from build123d import *

# Parameters (mm, degrees)
SKIZZE1_W                                   = 27
SKIZZE1_H                                   = 31
AUFSATZ_LINEAR_AUSTRAGEN1_DEPTH             = 20
AUFSATZ_LINEAR_AUSTRAGEN2_DEPTH             = 3
FORMSENKUNG_F_R_M3_SENKSCHRAUBE_MIT_2_COUNT = 2
FORMSENKUNG_F_R_M3_SENKSCHRAUBE_MIT_2_PITCH = 36
SCHNITT_LINEAR_AUSTRAGEN1_DEPTH             = 18
FASE1_SIZE                                  = 5
VERRUNDUNG1_R                               = 2


with BuildPart() as part:
    # Skizze1 → Aufsatz-Linear austragen1 (new body)
    with BuildSketch(Plane.XY):
        Rectangle(SKIZZE1_W, SKIZZE1_H)
    extrude(amount=AUFSATZ_LINEAR_AUSTRAGEN1_DEPTH)

    # Skizze2 → Aufsatz-Linear austragen2 (add)
    with BuildSketch(Plane.XY):
        Polygon((16.25, 17), (-16.25, 17), (-22.25, 9), (-22.25, -9), (-16.25, -17), (16.25, -17), (22.25, -9), (22.25, 9), align=None)
    extrude(amount=-AUFSATZ_LINEAR_AUSTRAGEN2_DEPTH)

    # Skizze3 → Formsenkung für M3 Senkschraube mit Innensechskant1 (revolve, cut)
    with BuildSketch(Plane(origin=(18, 0, -3), x_dir=(0, 1, 0), z_dir=(1, 0, 0))):
        Polygon((0, 0), (0, 3), (1.7, 3), (1.7, 1.77), (3.47, 0), align=None)
    formsenkung_f_r_m3_senkschraube_mit_inne = revolve(axis=Axis((18, 0, -9.35), (0, 0, 1)), mode=Mode.SUBTRACT)

    # Formsenkung f_r M3 Senkschraube mit  2: Formsenkung für M3 Senkschraube mit Innensechskant1 ×2
    with Locations(*[(-i * FORMSENKUNG_F_R_M3_SENKSCHRAUBE_MIT_2_PITCH, 0, 0) for i in range(1, FORMSENKUNG_F_R_M3_SENKSCHRAUBE_MIT_2_COUNT)]):
        add(formsenkung_f_r_m3_senkschraube_mit_inne, mode=Mode.SUBTRACT)

    # Skizze5 → Schnitt-Linear austragen1 (cut)
    with BuildSketch(Plane(origin=(0, 0, -3), x_dir=(-1, 0, 0), z_dir=(0, 0, -1))):
        Polygon((7.25, 14), (-7.25, 14), (-12.25, 9), (-12.25, -2), (12.25, -2), (12.25, 9), align=None)
    extrude(amount=-SCHNITT_LINEAR_AUSTRAGEN1_DEPTH, mode=Mode.SUBTRACT)

    # Fase1
    fase1_edges = [part.edges().sort_by_distance(p)[0] for p in [
        (-13.5, 15.5, 10),
        (13.5, 15.5, 10),
    ]]
    chamfer(fase1_edges, length=FASE1_SIZE)

    # Verrundung1
    verrundung1_edges = [part.edges().sort_by_distance(p)[0] for p in [
        (13.5, -15.5, 10),
        (-13.5, -15.5, 10),
    ]]
    fillet(verrundung1_edges, radius=VERRUNDUNG1_R)


solid = part.part
Design review of the part built by this model. Coordinates are the model's own, in mm. A direction names the side the tool comes from. Coordinates: 2 decimals unless noted, no trailing zeros. Order: outer loops, then holes, each group sorted by start corner. A loop starts at its lowest first (then second) coordinate and runs counter-clockwise, first axis right, second up. Notation, with made-up numbers: M 46.25,-19.5 L 74.25,-19.5 A18 ccw 74.25,8.5 Z; hole C -24,-10 d11. An arc over 180 degrees is marked long. Use a Markdown table: item, result.
(1) Draft analysis for pull direction Y (two halves, no side actions). For faces 5 (the cylindrical face through (12.9, -14.93, 10.14)), 6 (the flat face through (12.25, 4, 6)), 7 (the flat face through (11, 13, 10)), state which applies: released by +Y, released by -Y, zero draft, split by the parting line, or undercut.
Worked answers:
| item | result |
|---|---|
| face 5 | released by -Y |
| face 6 | undercut |
| face 7 | released by +Y |
(2) Add section D-D (y = -10). Give the boundary of the cut face in (x, z), then the cut area to 3 significant figures.
Worked answers:
| item | result |
|---|---|
| outline | M -21.5,-3 L 21.5,-3 L 21.5,0 L 13.5,0 L 13.5,20 L -13.5,20 L -13.5,0 L -21.5,0 Z |
| area | 669 mm2 |
(3) Add section C-C (x = -18). Give the boundary of the cut face in (y, z).
Worked answers:
| item | result |
|---|---|
| outline | M -14.67,-3 L -3.47,-3 L -1.7,-1.23 L -1.7,0 L -14.67,0 Z; M 1.7,-1.23 L 3.47,-3 L 14.67,-3 L 14.67,0 L 1.7,0 Z |
(4) For faces 1 (the flat face through (-12.25, 3, 6)), 2 (the flat face through (0, 15.5, 10)), 3 (the flat face through (-13.5, -2, 10)), 4 (the flat face through (-11, 13, 10)), list the 3-axis set-ups (+Z, -Z, +X, -X, +Y, -Y) from which the entire face can be reached by the end or side of a thin tool; tool diameter is ignored.
Worked answers:
| item | result |
|---|---|
| face 1 | -Z |
| face 2 | +Z, +X, -X, +Y |
| face 3 | +Z, -X, +Y, -Y |
| face 4 | +Z, -X, +Y |
(5) Add section A-A (y = 0). Give the boundary of the cut face in (x, z), then the cut area to 3 significant figures.
Worked answers:
| item | result |
|---|---|
| outline | M -22.25,-3 L -21.47,-3 L -19.7,-1.23 L -19.7,0 L -22.25,0 Z; M -16.3,-1.23 L -14.53,-3 L -12.25,-3 L -12.25,15 L 12.25,15 L 12.25,-3 L 14.53,-3 L 16.3,-1.23 L 16.3,0 L 13.5,0 L 13.5,20 L -13.5,20 L -13.5,0 L -16.3,0 Z; M 19.7,-1.23 L 21.47,-3 L 22.25,-3 L 22.25,0 L 19.7,0 Z |
| area | 206 mm2 |
(6) Wall thickness on probe 1 along X at (y, z) = (0, -0.75); probe 2 along X at (y, z) = (-1.5, 5.75); probe 3 along Y at (x, z) = (5.5, 1.25): over which ranges is each line inside the solid? List them lowest first.
Worked answers:
| item | result |
|---|---|
| probe 1 | x = -22.25 to -19.7, -16.3 to -12.25, 12.25 to 16.3, 19.7 to 22.25 |
| probe 2 | x = -13.5 to -12.25, 12.25 to 13.5 |
| probe 3 | y = -15.5 to -2, 14 to 15.5 |
(7) For P1, Ø5.5, axis at y = 4, z = 9.5, coming from the +X side; P2, Ø5.5, axis at y = 5, z = 3.5, coming from the -X side; P3, Ø4.5, axis at x = -18, y = 0, coming from the -Z side; P4, Ø2.5, axis at x = 18, y = 0, coming from the -Z side, all flat-tipped, find the tip position at first contact; note any pin that passes through.
Worked answers:
| item | result |
|---|---|
| P1 | stops at x = 13.5 |
| P2 | stops at x = -13.5 |
| P3 | stops at z = -1.78 |
| P4 | passes through |
(8) Add section B-B (z = 9.75). Give the boundary of the cut face in (x, y).
Worked answers:
| item | result |
|---|---|
| outline | M -13.5,-13.5 A2 ccw -11.5,-15.5 L 11.5,-15.5 A2 ccw 13.5,-13.5 L 13.5,10.5 L 8.5,15.5 L -8.5,15.5 L -13.5,10.5 Z; hole M -12.25,-2 L 12.25,-2 L 12.25,9 L 7.25,14 L -7.25,14 L -12.25,9 Z |
